Verification items for the finished model (mm, model axes). Face numbers are marked on the shaded views. A direction names the side the tool comes from. Round coordinates to 2 decimals unless told otherwise and drop trailing zeros. Order: outer loops, then holes, each group sorted by start corner. A loop starts at its lowest first (then second) coordinate and runs counter-clockwise, first axis right, second up. Notation, with made-up numbers: M 64,4 L 84,4 A26 cw 84,31 Z; hole C 58,72 d1. An arc over 180 degrees is marked long. Return JSON: item names as keys, results as strings. Group by question number.
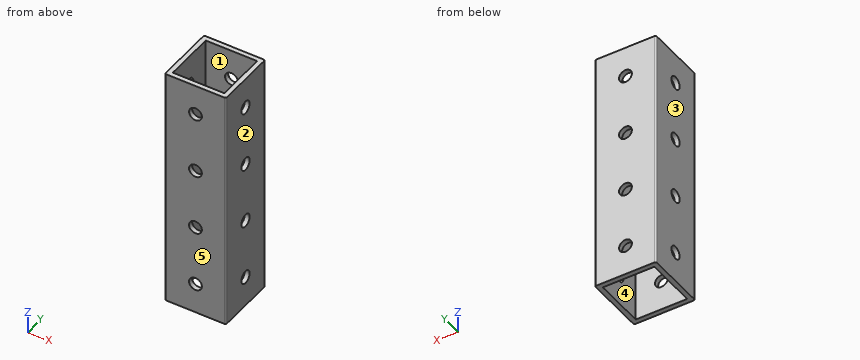
from build123d import *

# Parameters (mm, degrees)
BOX001_W               = 32.1
BOX001_H               = 32.1
BOX001_DEPTH           = 152.4
CYLINDER_R             = 4
CYLINDER_DEPTH         = 38.1
CYLINDER_PITCH_ANGLE   = 90
ARRAY001_Z_COUNT       = 4
ARRAY001_Z_PITCH       = 38.1
CYLINDER001_R          = 4
CYLINDER001_DEPTH      = 38.1
CYLINDER001_ROLL_ANGLE = 90
ARRAY_Z_COUNT          = 4
ARRAY_Z_PITCH          = 38.1
BOX_W                  = 38.1
BOX_H                  = 38.1
BOX_DEPTH              = 152.4
FILLET_R               = 1


with BuildPart() as cutout:
    # Box001 → Box001 (new body)
    with BuildSketch(Plane(origin=(3, 3, 0), x_dir=(1, 0, 0), z_dir=(0, 0, 1))):
        with Locations((16.05, 16.05)):
            Rectangle(BOX001_W, BOX001_H)
    extrude(amount=BOX001_DEPTH)


with BuildPart() as holes2:
    # Cylinder → Cylinder (new body)
    with BuildSketch(Plane.XY):
        Circle(CYLINDER_R)
    extrude(amount=CYLINDER_DEPTH)


with BuildPart() as holes2_1:
    # Cylinder pitch: moved
    add(holes2.part.rotate(Axis((0, 0, 0), (0, 1, 0)), CYLINDER_PITCH_ANGLE))


with BuildPart() as holes2_2:
    # Cylinder placement: moved
    add(holes2_1.part.moved(Location((0, 19.05, 19.05))))

    # Array001 Z: Holes2 ×4


with BuildPart() as holes2_3:
    add(holes2_2.part)
    with Locations(*[(0, 0, i * ARRAY001_Z_PITCH) for i in range(1, ARRAY001_Z_COUNT)]):
        add(holes2_2.part)


with BuildPart() as holes1:
    # Cylinder001 → Cylinder001 (new body)
    with BuildSketch(Plane.XY):
        Circle(CYLINDER001_R)
    extrude(amount=CYLINDER001_DEPTH)


with BuildPart() as holes1_1:
    # Cylinder001 roll: moved
    add(holes1.part.rotate(Axis((0, 0, 0), (1, 0, 0)), CYLINDER001_ROLL_ANGLE))


with BuildPart() as holes1_2:
    # Cylinder001 placement: moved
    add(holes1_1.part.moved(Location((19.05, 38.1, 19.05))))

    # Array Z: Holes1 ×4


with BuildPart() as holes1_3:
    add(holes1_2.part)
    with Locations(*[(0, 0, i * ARRAY_Z_PITCH) for i in range(1, ARRAY_Z_COUNT)]):
        add(holes1_2.part)


with BuildPart() as cut002:
    # Box → Box (new body)
    with BuildSketch(Plane.XY):
        with Locations((19.05, 19.05)):
            Rectangle(BOX_W, BOX_H)
    extrude(amount=BOX_DEPTH)

    # Fillet
    fillet_edges = [cut002.edges().sort_by_distance(p)[0] for p in [
        (0, 0, 76.2),
        (38.1, 0, 76.2),
        (38.1, 38.1, 76.2),
        (0, 38.1, 76.2),
    ]]
    fillet(fillet_edges, radius=FILLET_R)

    # Cut: cut Holes1
    add(holes1_3.part, mode=Mode.SUBTRACT)

    # Cut001: cut Holes2
    add(holes2_3.part, mode=Mode.SUBTRACT)

    # Cut002: cut Cutout
    add(cutout.part, mode=Mode.SUBTRACT)


solid = cut002.part
1. Cross-section at D-D (z = 35). Enter the section's corners in (x, y), plus the area to 3 significant figures.
2. Access from +Z, -Z, +X, -X, +Y, -Y to the whole of each face (thin tool, end or side, straight path). Record for the marked faces 1 and 2.
3. Thickness scan on line 1 along Z through (x, y) = (0.9, 19.05); line 2 along Y through (x, z) = (18, 8). Record the ranges inside material, lowest first. Write a range as from..to.
4. Cross-section at C-C (z = 95.25). Enter the section's corners in (x, y).
5. Cross-section at A-A (x = 27.5). Enter the section's corners in (y, z).
6. Draft check along Y on the marked faces 3, 4 and 5. Enter one of: +Y half, -Y half, draft (parallel to the pull), parting line (faces both ways), or undercut.
Computed:
{
 "1": {"outline": "M 0,1 A1 ccw 1,0 L 37.1,0 A1 ccw 38.1,1 L 38.1,37.1 A1 ccw 37.1,38.1 L 1,38.1 A1 ccw 0,37.1 Z; hole M 3,3 L 35.1,3 L 35.1,35.1 L 3,35.1 Z", "area": "420 mm²"},
 "2": {"face 1": "+Z, -Z", "face 2": "+Z, -Z, +X, +Y, -Y"},
 "3": {"line 1": "z = 0..15.05, 23.05..53.15, 61.15..91.25, 99.25..129.35, 137.35..152.4", "line 2": "y = 0..3, 35.1..38.1"},
 "4": {"outline": "M 0,1 A1 ccw 1,0 L 15.05,0 L 15.05,3 L 3,3 L 3,15.05 L 0,15.05 Z; M 0,23.05 L 3,23.05 L 3,35.1 L 15.05,35.1 L 15.05,38.1 L 1,38.1 A1 ccw 0,37.1 Z; M 23.05,0 L 37.1,0 A1 ccw 38.1,1 L 38.1,15.05 L 35.1,15.05 L 35.1,3 L 23.05,3 Z; M 23.05,35.1 L 35.1,35.1 L 35.1,23.05 L 38.1,23.05 L 38.1,37.1 A1 ccw 37.1,38.1 L 23.05,38.1 Z"},
 "5": {"outline": "M 0,0 L 3,0 L 3,152.4 L 0,152.4 Z; M 35.1,0 L 38.1,0 L 38.1,152.4 L 35.1,152.4 Z"},
 "6": {"face 3": "draft", "face 4": "undercut", "face 5": "-Y half"}
}
